```python
from build123d import *

# Parameters (mm, degrees)
EXTRUDE_1_DEPTH              = 45
CUT_EXTRUDE_1_DEPTH          = 26
SKETCH_4_R                   = 13
CUT_EXTRUDE_2_DEPTH          = 99.1035198
SKETCH_5_R                   = 13
CUT_EXTRUDE_3_DEPTH          = 6
SKETCH_7_W                   = 45.202600284
SKETCH_7_H                   = 48.529850946
CUT_EXTRUDE_4_DEPTH          = 131.224040013
SKETCH_8_R                   = 26
SKETCH_8_R_2                 = 11
EXTRUDE_3_DEPTH              = 15
HOLE_WIZARD_M5_1_D           = 4.2
HOLE_WIZARD_M5_1_DEPTH       = 12
HOLE_WIZARD_M5_1_CSINK_D     = 5.05
HOLE_WIZARD_M5_1_CSINK_ANGLE = 92
HOLE_WIZARD_M5_1_TIP         = 1.2618073
SKETCH_17_R                  = 3


with BuildPart() as part:
    # 스케치1 → 보스-돌출1 (new body)
    with BuildSketch(Plane.XY):
        with BuildLine():
            Line((5.476321218, 36.260519483), (20, 36.260519483))
            Line((20, 36.260519483), (20, 56.260519483))
            Line((20, 56.260519483), (44, 56.260519483))
            Line((44, 56.260519483), (44, -39.739480517))
            ThreePointArc((44, -39.739480517), (0, -83.739480517), (-44, -39.739480517))
            Line((-44, -39.739480517), (-44, 56.260519483))
            Line((-44, 56.260519483), (-20, 56.260519483))
            Line((-20, 56.260519483), (-20, 36.260519483))
            Line((-20, 36.260519483), (5.476321218, 36.260519483))
        make_face()
    extrude(amount=EXTRUDE_1_DEPTH)

    # 스케치3 → 컷-돌출1 (cut)
    with BuildSketch(Plane.XY.offset(45)):
        with BuildLine():
            Line((22, 0), (22, -40))
            ThreePointArc((22, -40), (0, -62), (-22, -40))
            Line((-22, -40), (-22, 0))
            ThreePointArc((-22, 0), (0, 22), (22, 0))
        make_face()
    extrude(amount=-CUT_EXTRUDE_1_DEPTH, mode=Mode.SUBTRACT)

    # 스케치4 → 컷-돌출2 (cut, through all)
    with BuildSketch(Plane.XY.offset(19)):
        Circle(SKETCH_4_R)
    extrude(amount=-CUT_EXTRUDE_2_DEPTH, mode=Mode.SUBTRACT)

    # 스케치5 → 컷-돌출3 (cut)
    with BuildSketch(Plane.XY.offset(19)):
        with Locations((0, -40)):
            Circle(SKETCH_5_R)
    extrude(amount=-CUT_EXTRUDE_3_DEPTH, mode=Mode.SUBTRACT)

    # 스케치7 → 컷-돌출4 (cut, through all)
    with BuildSketch(Plane(origin=(45, 0, 0), x_dir=(0, 0, -1), z_dir=(1, 0, 0))):
        with Locations((1.601300142, 60.525444956)):
            Rectangle(SKETCH_7_W, SKETCH_7_H)
    extrude(amount=-CUT_EXTRUDE_4_DEPTH, mode=Mode.SUBTRACT)

    # 스케치8 → 보스-돌출3 (add)
    with BuildSketch(Plane(origin=(0, 0, 0), x_dir=(-1, 0, 0), z_dir=(0, 0, -1))):
        Circle(SKETCH_8_R)
        Circle(SKETCH_8_R_2, mode=Mode.SUBTRACT)
    extrude(amount=EXTRUDE_3_DEPTH)

    # 스케치13 → M12x1.5 나사 구멍3 (revolve, cut)
    with BuildSketch(Plane(origin=(32, 56.260519483, 33), x_dir=(0, 0, 1), z_dir=(1, 0, 0))):
        Polygon((0, 0), (0, 21.15451825), (5.25, 18), (5.25, 0.7484088), (6.025, 0), align=None)
    m12x1_5_3 = revolve(axis=Axis((32, 62.610519483, 33), (0, -1, 0)), mode=Mode.SUBTRACT)

    # 대칭 복사1: M12x1.5 나사 구멍3 across plane
    add(m12x1_5_3.mirror(Plane(origin=(0, 0, 0), x_dir=(0, 0, 1), z_dir=(1, 0, 0))), mode=Mode.SUBTRACT)

    # M5 나사 구멍1
    with Locations(Plane(origin=(0, 29, 0), x_dir=(-1, 0, 0), z_dir=(0, 0, -1))):
        with Locations((0, 0), (0, -101)):
            CounterSinkHole(HOLE_WIZARD_M5_1_D / 2, HOLE_WIZARD_M5_1_CSINK_D / 2, depth=HOLE_WIZARD_M5_1_DEPTH, counter_sink_angle=HOLE_WIZARD_M5_1_CSINK_ANGLE)
            with Locations((0, 0, -(HOLE_WIZARD_M5_1_DEPTH + HOLE_WIZARD_M5_1_TIP / 2))):  # 118° drill point
                Cone(0, HOLE_WIZARD_M5_1_D / 2, HOLE_WIZARD_M5_1_TIP, mode=Mode.SUBTRACT)

    # 컷-스윕1: sweep along a path in 스케치16
    with BuildLine(Plane.XY.offset(33)) as sweep_1_path:
        Line((-32, 56.260519483), (-32, -13.739480517))
        ThreePointArc((-32, -13.739480517), (-30.242640687, -17.982121204), (-26, -19.739480517))
        Line((-26, -19.739480517), (-16.926354954, -19.739480517))
    # 스케치17 → 컷-스윕1 (sweep, cut)
    with BuildSketch(Plane(origin=(-32, 56.260519483, 33), x_dir=(-1, 0, 0), z_dir=(0, -1, 0))):
        Circle(SKETCH_17_R)
    sweep_1 = sweep(path=sweep_1_path.line, mode=Mode.SUBTRACT)

    # 대칭 복사3: 컷-스윕1 across plane
    add(sweep_1.mirror(Plane(origin=(0, 0, 0), x_dir=(0, 0, 1), z_dir=(1, 0, 0))), mode=Mode.SUBTRACT)


solid = part.part
```
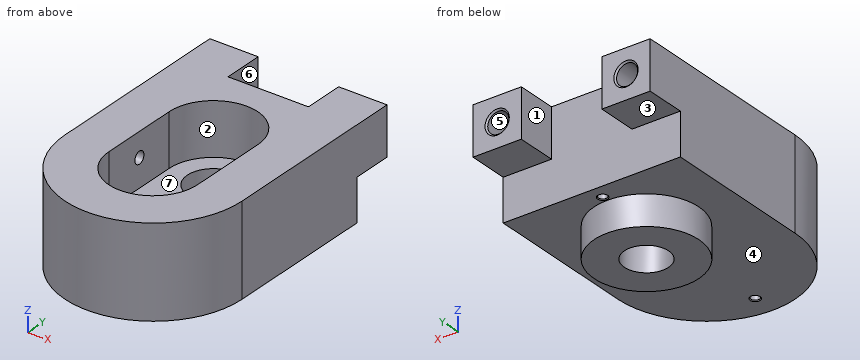
For this review, take the finished solid that the model builds, in its own axes (mm). Face numbers are marked on the shaded views. A direction names the side the tool comes from. Round coordinates to 2 decimals unless told otherwise and drop trailing zeros. Write each loop counter-clockwise with the first axis right and the second up, starting at its lowest first coordinate (ties: lowest second). Pieces come first, ordered by that corner, then holes. Notation, with made-up numbers: (-23, 60.25) -> (-4, 60.25) arc R8 cw to (-4, 68.25) -> close; hole circle Ø5 at (7, -21.5). An arc over 180 degrees is marked (long way). One line per question, with ' | ' between items. Start each with the question number.
1) Wall thickness on line 1 along Y through (x, z) = (0, 14.25); line 2 along X through (y, z) = (-2.5, 33); line 3 along Y through (x, z) = (0, 9): over which ranges is each line inside the solid? List them lowest first.
2) Mouldability with a two-part tool opening along Z and no side actions: class the marked faces 4, 5, 6 and 7 as +Z half, -Z half, draft (parallel to the pull), parting line (faces both ways), or undercut.
3) Add section B-B (y = -9). Write out the cut boundary in (x, z), and give its area (3 significant figures).
4) Machinability: for the marked faces 1, 2 and 3, which of the approach directions +Z, -Z, +X, -X, +Y, -Y give a long, thin tool a straight path to every point of the face, cutting with its end or side? Answer none if there is none.
5) Add section D-D (y = -37.5). Write out the cut boundary in (x, z).
6) For pin 1 Ø6 at (x, y) = (30.5, 41.5) entering from -Z; pin 2 Ø8.5 at (x, z) = (32, 33) entering from +Y; pin 3 Ø9.5 at (x, z) = (-32, 33) entering from +Y; pin 4 Ø3 at (x, z) = (29, -3) entering from +Y, all flat-tipped, find the tip position at first contact; note any pin that passes through.
7) Add section C-C (x = 16). Write out the cut boundary in (y, z), and give its area (3 significant figures).
8) Add section A-A (z = 5.5). Write out the cut boundary in (x, y).
Reported:
1) line 1: y = -83.74 to -53, -27 to -13, 13 to 36.26 | line 2: x = -44 to -35, -29 to -22, 22 to 29, 35 to 44 | line 3: y = -83.74 to -74.1, -69.9 to -13, 13 to 26.9, 31.1 to 36.26
2) face 4: -Z half | face 5: undercut | face 6: draft | face 7: +Z half
3) outline: (-44, 0) -> (-24.39, 0) -> (-24.39, -15) -> (-6.32, -15) -> (-6.32, 0) -> (-9.38, 0) -> (-9.38, 19) -> (-22, 19) -> (-22, 45) -> (-44, 45) -> close; (6.32, -15) -> (24.39, -15) -> (24.39, 0) -> (44, 0) -> (44, 45) -> (22, 45) -> (22, 19) -> (9.38, 19) -> (9.38, 0) -> (6.32, 0) -> close; hole circle Ø6 at (-32, 33); hole circle Ø6 at (32, 33) | area: 2,950 mm²
4) face 1: +Z, -Z, +Y | face 2: +Z | face 3: -Z, +X, -X, +Y
5) outline: (-44, 0) -> (44, 0) -> (44, 45) -> (22, 45) -> (22, 19) -> (12.76, 19) -> (12.76, 13) -> (-12.76, 13) -> (-12.76, 19) -> (-22, 19) -> (-22, 45) -> (-44, 45) -> close
6) pin 1: stops at z = 21 | pin 2: stops at y = 37.66 | pin 3: stops at y = 37.96 | pin 4: passes through
7) outline: (-80.73, 0) -> (-20.49, 0) -> (-20.49, -15) -> (20.49, -15) -> (20.49, 0) -> (36.26, 0) -> (36.26, 45) -> (15.1, 45) -> (15.1, 19) -> (-55.1, 19) -> (-55.1, 45) -> (-80.73, 45) -> close | area: 4,050 mm²
8) outline: (-44, -39.74) arc R44 ccw to (44, -39.74) -> (44, 36.26) -> (-44, 36.26) -> close; hole circle Ø26 at (0, 0); hole circle Ø4.2 at (0, -72); hole circle Ø4.2 at (0, 29)
